For this review, take the finished solid that the model builds, in its own axes (mm). A direction names the side the tool comes from. Give positions to 0.01 mm unless a question says otherwise; leave off trailing zeros. Write each loop counter-clockwise with the first axis right and the second up, starting at its lowest first coordinate (ties: lowest second). Pieces come first, ordered by that corner, then holes. Notation, with made-up numbers: (-17.5, 24) -> (36.5, 24) arc R34 ccw to (36.5, 60) -> close; hole circle Ø11 at (-36.5, 77.25). An arc over 180 degrees is marked (long way). Answer as CSV lines item,"result".
```python
from build123d import *

# Parameters (mm, degrees)
SKETCH1_R           = 11.65
SKETCH1_R_2         = 1.15
BOSS_EXTRUDE1_DEPTH = 8.5
SKETCH3_R           = 11.65
SKETCH3_R_2         = 9.65
BOSS_EXTRUDE3_DEPTH = 4.5
FILLET2_R           = 2


with BuildPart() as part:
    # Sketch1 → Boss-Extrude1 (new body)
    with BuildSketch(Plane(origin=(0, 0, 0), x_dir=(1, 0, 0), z_dir=(0, 1, 0))):
        with Locations(Location((0, 0, 0), (0, 0, 270))):
            Circle(SKETCH1_R)
        with Locations(Location((-3.5, 3.5, 0), (0, 0, 270))):
            Circle(SKETCH1_R_2, mode=Mode.SUBTRACT)
        with Locations(Location((3.5, 3.5, 0), (0, 0, 270))):
            Circle(SKETCH1_R_2, mode=Mode.SUBTRACT)
        with Locations(Location((3.5, -3.5, 0), (0, 0, 270))):
            Circle(SKETCH1_R_2, mode=Mode.SUBTRACT)
        with Locations(Location((-3.5, -3.5, 0), (0, 0, 270))):
            Circle(SKETCH1_R_2, mode=Mode.SUBTRACT)
    extrude(amount=BOSS_EXTRUDE1_DEPTH)

    # Sketch3 → Boss-Extrude3 (add)
    with BuildSketch(Plane(origin=(0, 8.5, 0), x_dir=(1, 0, 0), z_dir=(0, 1, 0))):
        with Locations(Location((0, 0, 0), (0, 0, 270))):
            Circle(SKETCH3_R)
        with Locations(Location((0, 0, 0), (0, 0, 270))):
            Circle(SKETCH3_R_2, mode=Mode.SUBTRACT)
    extrude(amount=BOSS_EXTRUDE3_DEPTH)

    # Fillet2
    fillet2_edges = [part.edges().sort_by_distance(p)[0] for p in [
        (0, 8.5, -9.65),
    ]]
    fillet(fillet2_edges, radius=FILLET2_R)


solid = part.part
```
Q1. Draft analysis for pull direction X (two halves, no side actions). For faces 1 (the flat face through (9, 13, -4)), 2 (the cylindrical face through (-2.723, 4.19, -4.348)), 3 (the cylindrical face through (-11.37, 6.41, -2.53)), state which applies: released by +X, released by -X, zero draft, split by the parting line, or undercut.
Answer block:
face 1,"zero draft"
face 2,"undercut"
face 3,"split by the parting line"
Q2. To check wall thickness, follow probe 1 along X at (y, z) = (12.3, 0); probe 2 along X at (y, z) = (3.25, 2.5); probe 3 along X at (y, z) = (3.25, -3.5). State the ranges of each line that lie inside material, in increasing order. Write a range as [from, to].
Answer block:
probe 1,"x = [-11.65, -9.65], [9.65, 11.65]"
probe 2,"x = [-11.38, -4.07], [-2.93, 2.93], [4.07, 11.38]"
probe 3,"x = [-11.11, -4.65], [-2.35, 2.35], [4.65, 11.11]"
Q3. For faces 4 (the cylindrical face through (9.568, 11.732, -1.256)), 5 (the flat face through (0, 0, 0)), list the 3-axis set-ups (+Z, -Z, +X, -X, +Y, -Y) from which the entire face can be reached by the end or side of a thin tool; tool diameter is ignored.
Answer block:
face 4,"+Y"
face 5,"+Z, -Z, +X, -X, -Y"
Q4. Add section D-D (y = 12). Write out the cut boundary in (x, z).
Answer block:
outline,"circle Ø23.3 at (0, 0); hole circle Ø19.3 at (0, 0)"
Q5. Clearance check with flat-ended pins moving along their axes: pin 1 (1.4 mm diameter, centred on x = -3.5, z = 3.5, fed in from +Y); pin 2 (4 mm diameter, centred on y = 9.5, z = -4.5, fed in from -X); pin 3 (5 mm diameter, centred on x = -1.5, z = 5, fed in from +Y); pin 4 (2 mm diameter, centred on x = 7, y = 5.5, fed in from +Z). State where each tip first meets the part, or that it passes through.
Answer block:
pin 1,"passes through"
pin 2,"stops at x = -11.38"
pin 3,"stops at y = 8.5"
pin 4,"stops at z = 9.99"
Q6. Add section C-C (z = 0). Write out the cut boundary in (x, y), plus the area to 3 significant figures.
Answer block:
outline,"(-11.65, 0) -> (11.65, 0) -> (11.65, 13) -> (9.65, 13) -> (9.65, 10.5) arc R2 cw to (7.65, 8.5) -> (-7.65, 8.5) arc R2 cw to (-9.65, 10.5) -> (-9.65, 13) -> (-11.65, 13) -> close"
area,"218 mm2"
Q7. Add section B-B (x = 0). Write out the cut boundary in (y, z).
Answer block:
outline,"(0, -11.65) -> (13, -11.65) -> (13, -9.65) -> (10.5, -9.65) arc R2 cw to (8.5, -7.65) -> (8.5, 7.65) arc R2 cw to (10.5, 9.65) -> (13, 9.65) -> (13, 11.65) -> (0, 11.65) -> close"
Q8. Add section A-A (y = 1.5). Write out the cut boundary in (x, z), plus the area to 3 significant figures.
Answer block:
outline,"circle Ø23.3 at (0, 0); hole circle Ø2.3 at (-3.5, -3.5); hole circle Ø2.3 at (-3.5, 3.5); hole circle Ø2.3 at (3.5, -3.5); hole circle Ø2.3 at (3.5, 3.5)"
area,"410 mm2"
